Verification items for this drawing (mm, ordinates from the low corner). Give positions to 0.01 mm unless a question says otherwise; leave off trailing zeros. Write each loop counter-clockwise with the first axis right and the second up, starting at its lowest first coordinate (ties: lowest second). Pieces come first, ordered by that corner, then holes. Notation, with made-up numbers: (54.5, -14.5) -> (95.5, -14.5) arc R17 ccw to (95.5, -7.5) -> close; hole circle Ø1 at (65, 33.25). An arc over 180 degrees is marked (long way). Answer as a JSON object with one key per item and string values.
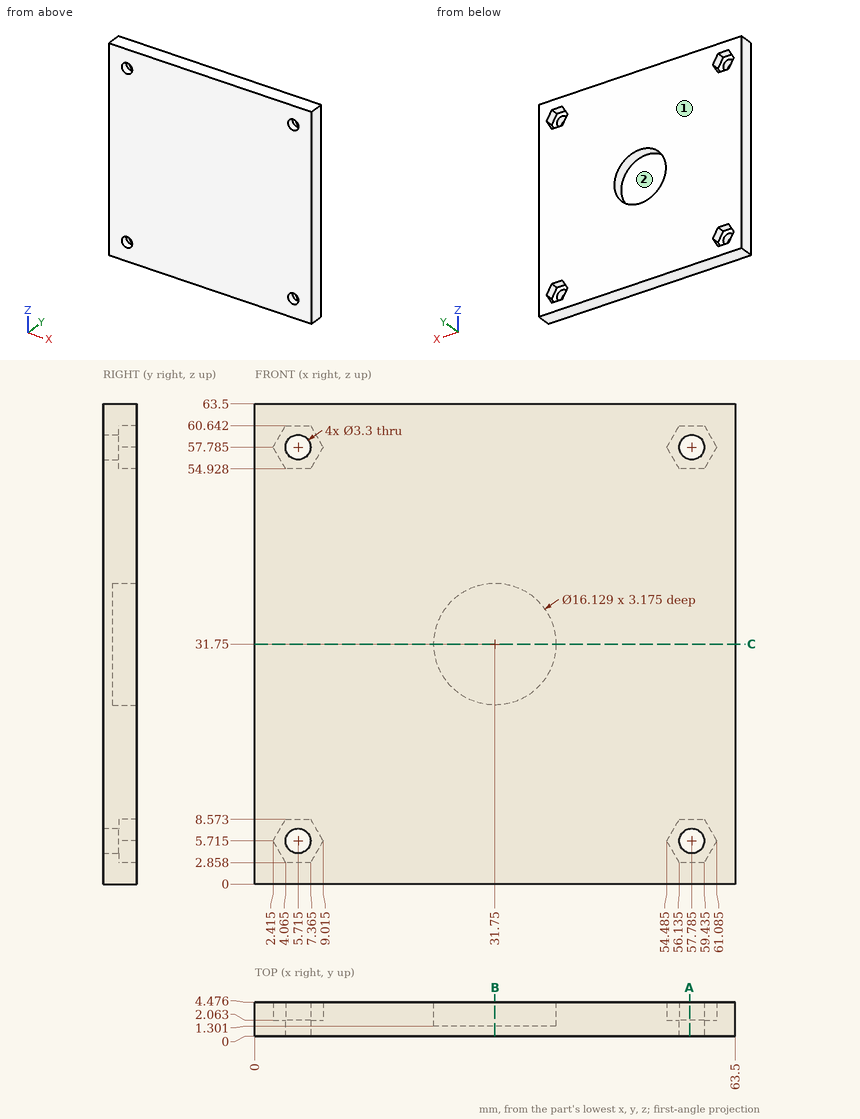
1. Sectioned sample at C-C, the plane z = 31.75. Enter the section's corners in (x, y) (1 decimal), plus the area to 3 significant figures.
Determined:
{"outline": "(0, 0) -> (63.5, 0) -> (63.5, 4.5) -> (39.8, 4.5) -> (39.8, 1.3) -> (23.7, 1.3) -> (23.7, 4.5) -> (0, 4.5) -> close", "area": "233 mm^2"}
2. Mould release check, pull along X, two halves, no side actions. Record for the marked faces 1 and 2: released by +X, released by -X, zero draft, split by the parting line, or undercut.
Determined:
{"face 1": "zero draft", "face 2": "undercut"}
3. Sectioned sample at B-B, the plane x = 31.75. Enter the section's corners in (y, z) (1 decimal).
Determined:
{"outline": "(0, 0) -> (4.5, 0) -> (4.5, 23.7) -> (1.3, 23.7) -> (1.3, 39.8) -> (4.5, 39.8) -> (4.5, 63.5) -> (0, 63.5) -> close"}
4. Sectioned sample at A-A, the plane x = 57.5. Enter the section's corners in (y, z) (1 decimal), plus the area to 3 significant figures.
Determined:
{"outline": "(0, 0) -> (4.5, 0) -> (4.5, 2.9) -> (2.1, 2.9) -> (2.1, 4.1) -> (0, 4.1) -> close; (0, 7.3) -> (2.1, 7.3) -> (2.1, 8.6) -> (4.5, 8.6) -> (4.5, 54.9) -> (2.1, 54.9) -> (2.1, 56.2) -> (0, 56.2) -> close; (0, 59.4) -> (2.1, 59.4) -> (2.1, 60.6) -> (4.5, 60.6) -> (4.5, 63.5) -> (0, 63.5) -> close", "area": "243 mm^2"}
5. Scan lines: L1, parallel to Z at x = 57, y = 1.25 (1 decimal); L2, parallel to Z at x = 7, y = 1.05; L3, parallel to Z at x = 31.75, y = 2.6 (1 decimal). Record each from-to range of solid material in increasing order. Write a range as [from, to].
Determined:
{"L1": "[0, 4.3], [7.2, 56.3], [59.2, 63.5]", "L2": "[0, 4.68], [6.75, 56.75], [58.82, 63.5]", "L3": "[0, 23.7], [39.8, 63.5]"}
